Could you check a few things on this model? Use its own coordinates, in mm. Give positions to 0.01 mm unless a question says otherwise; leave off trailing zeros. Loops run counter-clockwise (first coordinate to the right, second up) from the corner with the lowest first, then second, coordinate; pieces in that order, holes last. Notation, with made-up numbers: M -22,-24 L -2,-24 A31 ccw -2,8 Z; hole C 88,17 d8. An arc over 180 degrees is marked long. Return JSON: item names as keys, results as strings. Group by question number.
1. For pin 1 (5 mm diameter, centred on y = 8.5, z = 291.5, fed in from +X); pin 2 (10 mm diameter, centred on x = -4.5, z = 130, fed in from -Y); pin 3 (3 mm diameter, centred on y = 6, z = 174.5, fed in from -X), each with a flat end and sliding along its axis, tell me the tip position at first contact or that it passes through.
2. If we section it at A-A (z = 308): Write out the boundary of the cut face in (x, y), plus the area to 3 significant figures.
3. Please list where these lines run through material, in increasing order: line 1 (Y direction, x = 0.5, z = 626.5); line 2 (Z direction, x = 85, y = -9.5); line 3 (Y direction, x = 23, z = 197).
4. If we section it at B-B (z = 767.5): Write out the boundary of the cut face in (x, y).
```python
from build123d import *

# Parameters (mm, degrees)
F0_R     = 85
F2_R     = 0.5
F4_R     = 105.9677495378
F5_DEPTH = 1


# Not quite as in the source:
# - a fillet or chamfer that OpenCascade refuses, or shapes differently, is made with other operations: its cross-section is extruded or revolved along the edge and cut away or added


with BuildPart() as f3:
    # F0 (on Top) → F3 section 0
    with BuildSketch(Plane.XY):
        Circle(F0_R)
    # F2 (on offset) → F3 section 1
    with BuildSketch(Plane.XY.offset(900)):
        Circle(F2_R)
    loft()

    # F4 (on Top) → F5 (join)
    with BuildSketch(Plane.XY):
        Circle(F4_R)
    extrude(amount=F5_DEPTH)

    # F6: fillet of radius 50 on 1 edges, made by hand


with BuildPart() as f6_tool2:
    # F6_s3 → F6_t4 (revolve)
    with BuildSketch(Plane.XZ):
        with BuildLine():
            ThreePointArc((105.9675487491, 0.9996540464), (88.9507928559, 17.2936216176), (81.2843067656, 39.5711518076))
            Line((81.2843067656, 39.5711518076), (76.3060471064, 39.1037485396))
            ThreePointArc((76.3060471064, 39.1037485396), (78.1171484035, 19.8181913314), (79.927851452, 0.532596732))
            Line((79.927851452, 0.532596732), (84.9061111111, -4.0001535025))
            ThreePointArc((84.9061111111, -4.0001535025), (95.4368299301, -4.0001535025), (103.4576132883, -3.3248989977))
            Line((103.4576132883, -3.3248989977), (105.9675487491, 0.9996540464))
        make_face()
    revolve(axis=Axis((0, 0, 1), (0, 0, 1)))

    split(bisect_by=Plane.XY, keep=Keep.TOP)


with BuildPart() as f3_1:
    add(f3.part)

    # F6_t1: union F6_tool2
    add(f6_tool2.part)


solid = f3_1.part
```
Answer:
{
 "1": {"pin 1": "stops at x = 57.41", "pin 2": "stops at y = -73.18", "pin 3": "stops at x = -68.54"},
 "2": {"outline": "C 0,0 d112.16", "area": "9,880 mm²"},
 "3": {"line 1": "y = -26.17 to 26.17", "line 2": "z = 0 to 23.59", "line 3": "y = -62.4 to 62.4"},
 "4": {"outline": "C 0,0 d25.88"}
}
